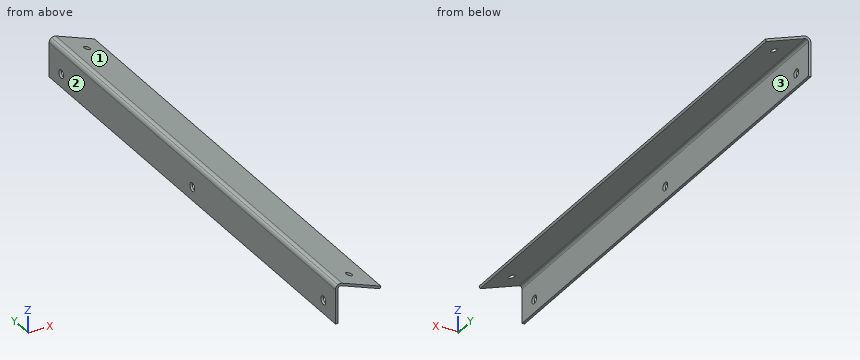
```python
from build123d import *

# Parameters (mm, degrees)
SKETCH1_W                = 300
SKETCH1_H                = 50
BASE_FLANGE1_DEPTH       = 1.5
SKETCHED_START           = -150
SKETCHED_BEND1_DEPTH     = 300
SKETCHED_BEND1_2_DEPTH   = 300
F_4_0_4_DIAMETER_HOLE1_D = 4
F_5_0_5_DIAMETER_HOLE1_D = 5


# Read off the part's stored shape, not the designer's step: Sketched Bend1
# Sheet-metal steps are written as plain solids
with BuildPart() as part:
    # Sketch1 → Base-Flange1 (new body)
    with BuildSketch(Plane.YZ):
        Rectangle(SKETCH1_W, SKETCH1_H)
    extrude(amount=-BASE_FLANGE1_DEPTH)

    # Sketched Bend1 outline → Sketched Bend1 (cut)
    with BuildSketch(Plane(origin=(0, 0, 0), x_dir=(1, 0, 0), z_dir=(0, 1, 0)).offset(SKETCHED_START)):
        with BuildLine():
            Line((0, -25), (0, 1.686367809))
            ThreePointArc((0, 1.686367809), (-1.098076211, 2.78444402), (-1.5, 4.28444402))
            Line((-1.5, 4.28444402), (-1.5, -25))
            Line((-1.5, -25), (0, -25))
        make_face()
    extrude(amount=SKETCHED_BEND1_DEPTH, mode=Mode.SUBTRACT)

    # Sketched Bend1 2 outline → Sketched Bend1 2 (add)
    with BuildSketch(Plane(origin=(0, 0, 0), x_dir=(1, 0, 0), z_dir=(0, 1, 0)).offset(SKETCHED_START)):
        with BuildLine():
            Line((25.472225443, 11.413353872), (2.013030215, 2.874905089))
            ThreePointArc((2.013030215, 2.874905089), (0.639635346, 3.055715954), (0, 4.28444402))
            Line((0, 4.28444402), (0, 1.686367809))
            ThreePointArc((0, 1.686367809), (1.238532772, 1.295859926), (2.52606043, 1.465366158))
            Line((2.52606043, 1.465366158), (25.985255658, 10.003814941))
            Line((25.985255658, 10.003814941), (25.472225443, 11.413353872))
        make_face()
    extrude(amount=SKETCHED_BEND1_2_DEPTH)

    # Ø4.0 (4) Diameter Hole1 (through all)
    with Locations(Plane(origin=(-0.175466668, 0, -0.482090707), x_dir=(0, -1, 0), z_dir=(0.3420201433256727, 0, 0.9396926207859071))):
        with Locations((-137.3, 15.139659211), (137.3, 15.139659211)):
            Hole(F_4_0_4_DIAMETER_HOLE1_D / 2)

    # Ø5.0 (5) Diameter Hole1 (through all)
    with Locations(Plane(origin=(-1.5, 0, 0), x_dir=(0, -1, 0), z_dir=(-1, 0, 0))):
        with Locations((-137.3, -16.98444402), (137.3, -16.98444402), (0, -16.98444402)):
            Hole(F_5_0_5_DIAMETER_HOLE1_D / 2)


solid = part.part
```
The model under review builds one solid part; all positions refer to its coordinate system, in mm. Face numbers are marked on the shaded views. Give positions to 0.01 mm unless a question says otherwise; leave off trailing zeros. Write each loop counter-clockwise with the first axis right and the second up, starting at its lowest first coordinate (ties: lowest second). Pieces come first, ordered by that corner, then holes. Notation, with made-up numbers: (-2, 21) - (50, 21) arc R24 ccw to (50, 42) - close; hole circle Ø7 at (24, 1). An arc over 180 degrees is marked (long way). Answer in a Markdown table with one row per item. Add a question column.
1. Insertion check: P1, Ø12, axis at x = 19.5, y = 110.5, coming from the +Z side; P2, Ø1, axis at x = 4.5, y = 104.5, coming from the -Z side; P3, Ø5, axis at x = 7.5, y = -105, coming from the -Z side; P4, Ø2, axis at x = 7, z = -7.5, coming from the +Y side. Each pin has a flat end and moves straight along its axis. Give the tip position at first contact, or say it passes through.
2. We need section C-C on x = 20.5. Write out the cut boundary in (y, z).
3. We need section A-A on y = 0. Write out the cut boundary in (x, z).
4. We need section B-B on y = -82. Write out the cut boundary in (x, z), then the cut area to 3 significant figures.
5. Draft analysis for pull direction X (two halves, no side actions). For the marked faces 1, 2 and 3, state which applies: +X half, -X half, draft (parallel to the pull), parting line (faces both ways), or undercut.
6. Wall thickness on line 1 along Z through (x, y) = (-0.95, 137.3); line 2 along X through (y, z) = (-75, -12.75); line 3 along Z through (x, y) = (-1.15, 137.3): over which ranges is each line inside the solid? List them lowest first. Write a range as [from, to].
Ans:
| question | item | result |
|---|---|---|
| 1 | P1 | stops at z = -5.46 |
| 1 | P2 | stops at z = -3.96 |
| 1 | P3 | stops at z = -5.78 |
| 1 | P4 | passes through |
| 2 | outline | (-150, -9.6) - (150, -9.6) - (150, -8.01) - (-150, -8.01) - close |
| 3 | outline | (-1.5, -25) - (0, -25) - (0, -19.48) - (-1.5, -19.48) - close; (-1.5, -14.48) - (0, -14.48) - (0, -4.28) arc R1.5 cw to (2.01, -2.87) - (25.47, -11.41) - (25.99, -10) - (2.53, -1.47) arc R3 ccw to (-1.5, -4.28) - close |
| 4 | outline | (-1.5, -25) - (0, -25) - (0, -4.28) arc R1.5 cw to (2.01, -2.87) - (25.47, -11.41) - (25.99, -10) - (2.53, -1.47) arc R3 ccw to (-1.5, -4.28) - close |
| 4 | area | 75.0 mm^2 |
| 5 | face 1 | +X half |
| 5 | face 2 | -X half |
| 5 | face 3 | undercut |
| 6 | line 1 | z = [-25, -19.48], [-14.48, -2.55] |
| 6 | line 2 | x = [-1.5, 0] |
| 6 | line 3 | z = [-25, -19.48], [-14.48, -2.88] |
